Geometry: final body of the model. Coordinates: model frame, mm. Face numbers are marked on the shaded views. A direction names the side the tool comes from. Round coordinates to 2 decimals unless told otherwise and drop trailing zeros. Loops run counter-clockwise (first coordinate to the right, second up) from the corner with the lowest first, then second, coordinate; pieces in that order, holes last. Notation, with made-up numbers: (-19.75, 64.25) - (-12.75, 64.25) arc R36 ccw to (-12.75, 98.25) - close; hole circle Ø11 at (32.25, 71). An arc over 180 degrees is marked (long way). Answer as CSV lines item,"result".
from build123d import *

# Parameters (mm, degrees)
SKETCH1_W           = 28.59
SKETCH1_H           = 20
BOSS_EXTRUDE1_DEPTH = 3
SKETCH2_W           = 3
SKETCH2_H           = 20
BOSS_EXTRUDE2_DEPTH = 6.175
BOSS_EXTRUDE3_DEPTH = 20
SKETCH5_W           = 5
SKETCH5_H           = 20
BOSS_EXTRUDE4_DEPTH = 10
BOSS_EXTRUDE5_DEPTH = 1.5
BOSS_EXTRUDE6_START = -1.5
BOSS_EXTRUDE6_DEPTH = 1.5
CUT_EXTRUDE1_START  = -20
SKETCH8_R           = 1.5
CUT_EXTRUDE1_DEPTH  = 20
SKETCH9_W           = 19.175
SKETCH9_H           = 17
CUT_EXTRUDE2_DEPTH  = 1
FILLET1_R           = 10
FILLET2_R           = 10
FILLET3_R           = 3


with BuildPart() as part:
    # Sketch1 → Boss-Extrude1 (new body)
    with BuildSketch(Plane.XY.offset(24.175)):
        with Locations((0, 65.691967044)):
            Rectangle(SKETCH1_W, SKETCH1_H)
    extrude(amount=BOSS_EXTRUDE1_DEPTH)

    # Sketch2 → Boss-Extrude2 (add)
    with BuildSketch(Plane(origin=(0, 0, 24.175), x_dir=(-1, 0, 0), z_dir=(0, 0, -1))):
        with Locations((-12.795, 65.691967044)):
            Rectangle(SKETCH2_W, SKETCH2_H)
        with Locations((12.795, 65.691967044)):
            Rectangle(SKETCH2_W, SKETCH2_H)
    extrude(amount=BOSS_EXTRUDE2_DEPTH)

    # Sketch4 → Boss-Extrude3 (add)
    with BuildSketch(Plane(origin=(0, 75.691967044, 0), x_dir=(1, 0, 0), z_dir=(0, 1, 0))):
        Polygon((-11.295, -20), (-11.295, -18), (-9.795, -20), align=None)
        Polygon((11.295, -18), (11.295, -20), (9.795, -20), align=None)
    extrude(amount=-BOSS_EXTRUDE3_DEPTH)

    # Sketch5 → Boss-Extrude4 (add)
    with BuildSketch(Plane.XY.offset(27.175)):
        with Locations((11.795, 65.691967044)):
            Rectangle(SKETCH5_W, SKETCH5_H)
    extrude(amount=BOSS_EXTRUDE4_DEPTH)

    # Sketch6 → Boss-Extrude5 (add)
    with BuildSketch(Plane.XZ.offset(-55.691967044)):
        with BuildLine():
            Line((11.295, 18), (11.795, 15.5))
            ThreePointArc((11.795, 15.5), (16.062766953, 13.732233047), (14.295, 18))
            Line((14.295, 18), (11.295, 18))
        make_face()
    extrude(amount=-BOSS_EXTRUDE5_DEPTH)

    # Sketch7 → Boss-Extrude6 (add)
    with BuildSketch(Plane(origin=(0, 75.691967044, 0), x_dir=(1, 0, 0), z_dir=(0, 1, 0)).offset(BOSS_EXTRUDE6_START)):
        with BuildLine():
            Line((11.295, -18), (11.795, -15.5))
            ThreePointArc((11.795, -15.5), (16.062766953, -13.732233047), (14.295, -18))
            Line((14.295, -18), (11.295, -18))
        make_face()
    extrude(amount=BOSS_EXTRUDE6_DEPTH)

    # Sketch8 → Cut-Extrude1 (cut)
    with BuildSketch(Plane(origin=(0, 75.691967044, 0), x_dir=(1, 0, 0), z_dir=(0, 1, 0)).offset(CUT_EXTRUDE1_START)):
        with Locations(Location((14.295, -15.5, 0), (0, 0, 270))):
            Circle(SKETCH8_R)
    extrude(amount=CUT_EXTRUDE1_DEPTH, mode=Mode.SUBTRACT)

    # Sketch9 → Cut-Extrude2 (cut)
    with BuildSketch(Plane(origin=(14.295, 0, 0), x_dir=(0, 0, -1), z_dir=(1, 0, 0))):
        with Locations((-27.5875, 65.691967044)):
            Rectangle(SKETCH9_W, SKETCH9_H)
    extrude(amount=-CUT_EXTRUDE2_DEPTH, mode=Mode.SUBTRACT)

    # Fillet1
    fillet1_edges = [part.edges().sort_by_distance(p)[0] for p in [
        (14.295, 74.941967044, 18),
        (14.295, 56.441967044, 18),
    ]]
    fillet(fillet1_edges, radius=FILLET1_R)

    # Fillet2
    fillet2_edges = [part.edges().sort_by_distance(p)[0] for p in [
        (11.295, 74.941967044, 18),
        (11.295, 56.441967044, 18),
    ]]
    fillet(fillet2_edges, radius=FILLET2_R)

    # Fillet3
    fillet3_edges = [part.edges().sort_by_distance(p)[0] for p in [
        (-14.295, 65.691967044, 27.175),
        (9.295, 65.691967044, 27.175),
        (9.295, 65.691967044, 37.175),
    ]]
    fillet(fillet3_edges, radius=FILLET3_R)


solid = part.part
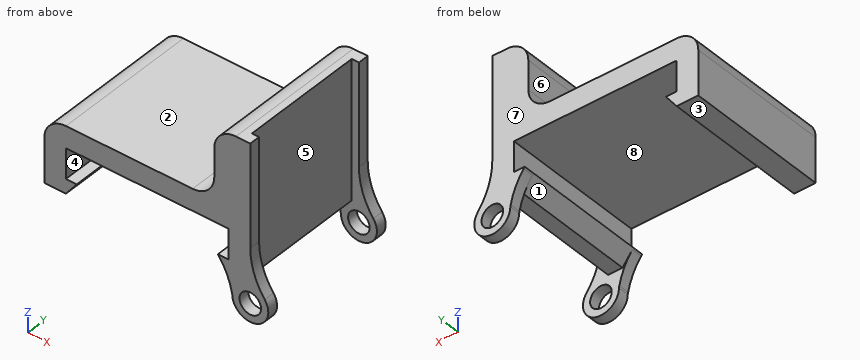
(1) Section B-B (y = 62.5). Output: boundary loops of the cut face in (x, z) (3 decimals), and give its area (3 significant figures).
Findings below:
outline,"(-14.295, 18) - (-11.295, 18) - (-9.795, 20) - (-11.295, 20) - (-11.295, 24.175) - (11.295, 24.175) - (11.295, 20) - (9.795, 20) - (11.295, 18) - (13.295, 18) - (13.295, 37.175) - (12.295, 37.175) arc R3 ccw to (9.295, 34.175) - (9.295, 30.175) arc R3 cw to (6.295, 27.175) - (-11.295, 27.175) arc R3 ccw to (-14.295, 24.175) - close"
area,"155 mm2"
(2) Access query for the marked faces 1, 2, 3 and 4. Directions: +Z, -Z, +X, -X, +Y, -Y. A direction counts if a zero-diameter tool reaches every point of the face in a straight line with its end or side. Return the directions, or none.
Findings below:
face 1,"-Z"
face 2,"+Z, -X, +Y, -Y"
face 3,"-Z, -X, +Y, -Y"
face 4,"+Y, -Y"
(3) Pin query (flat end, axial travel): P1, Ø6, axis at x = 4.5, y = 66.5, coming from the -Z side (3 decimals); P2, Ø1.8, axis at x = 14.295, z = 15.5, coming from the -Y side; P3, Ø3, axis at x = 10.5, y = 59.5, coming from the +Z side; P4, Ø1.5, axis at y = 59.5, z = 26, coming from the -X side. Return the tip coordinate at first contact, or that it passes through.
Findings below:
P1,"z = 24.175"
P2,"through"
P3,"z = 37.16"
P4,"x = -14.1"
(4) Draft query along X for the marked faces 5, 6, 7 and 8. Return one class per face: pulls with the +X half, pulls with the -X half, needs draft (parallel to the pull), parting line crosses it, or undercut.
Findings below:
face 5,"pulls with the +X half"
face 6,"pulls with the -X half"
face 7,"needs draft"
face 8,"undercut"
(5) Section D-D (x = 2). Output: boundary loops of the cut face in (y, z) (3 decimals).
Findings below:
outline,"(55.692, 24.175) - (75.692, 24.175) - (75.692, 27.175) - (55.692, 27.175) - close"
(6) Section A-A (z = 21.25). Output: boundary loops of the cut face in (x, y) (3 decimals), and give its area (3 significant figures).
Findings below:
outline,"(-14.295, 55.692) - (-11.295, 55.692) - (-11.295, 75.692) - (-14.295, 75.692) - close; (11.295, 55.692) - (14.449, 55.692) - (14.449, 57.192) - (13.295, 57.192) - (13.295, 74.192) - (14.449, 74.192) - (14.449, 75.692) - (11.295, 75.692) - close"
area,"103 mm2"
(7) Material intervals for line 1 along X through (y, z) = (56.5, 15.5) (3 decimals); line 2 along X through (y, z) = (63.25, 30) (3 decimals); line 3 along Z through (x, y) = (-3, 58.25) (3 decimals), sorted ascending.
Findings below:
line 1,"11.795 to 12.795, 15.795 to 16.795"
line 2,"9.29 to 13.295"
line 3,"24.175 to 27.175"
(8) Section C-C (z = 16.5). Output: boundary loops of the cut face in (x, y).
Findings below:
outline,"(11.57, 55.69) - (13.18, 55.69) - (13.18, 57.19) - (11.57, 57.19) - close; (11.57, 74.19) - (13.18, 74.19) - (13.18, 75.69) - (11.57, 75.69) - close; (15.41, 55.69) - (16.59, 55.69) - (16.59, 57.19) - (15.41, 57.19) - close; (15.41, 74.19) - (16.59, 74.19) - (16.59, 75.69) - (15.41, 75.69) - close"
